Input: part model. Units: mm. Frame: model coordinates. A direction names the side the tool comes from. Give positions to 0.01 mm unless a question says otherwise; leave off trailing zeros. Order: outer loops, then holes, each group sorted by start corner. A loop starts at its lowest first (then second) coordinate and runs counter-clockwise, first axis right, second up. Notation, with made-up numbers: M 11.5,58.5 L 51.5,58.5 A35 cw 51.5,96.5 Z; hole C 82.5,39.25 d1. An arc over 180 degrees is marked long. Use a Markdown table: item, result.
from build123d import *

# Parameters (mm, degrees)
SKETCH4_R           = 2.54
BOSS_EXTRUDE1_DEPTH = 1.27
SKETCH5_W           = 12.7
SKETCH5_H           = 1.27
BOSS_EXTRUDE2_DEPTH = 28.956


with BuildPart() as part:
    # Sketch4 → Boss-Extrude1 (new body)
    with BuildSketch(Plane.XY):
        Polygon((0, 0), (12.7, 0), (12.7, 20.32), (9.525, 23.609765797), (3.175, 23.609765797), (0, 20.32), align=None)
        with Locations((6.35, 18.246144904)):
            Circle(SKETCH4_R, mode=Mode.SUBTRACT)
    boss_extrude1 = extrude(amount=BOSS_EXTRUDE1_DEPTH)

    # Sketch5 → Boss-Extrude2 (add)
    with BuildSketch(Plane.XY.offset(1.27)):
        with Locations((6.35, 0.635)):
            Rectangle(SKETCH5_W, SKETCH5_H)
    extrude(amount=BOSS_EXTRUDE2_DEPTH)

    # Mirror1: Boss-Extrude1 across plane
    add(boss_extrude1.mirror(Plane.XY.offset(15.113)))


solid = part.part
1) Cut plane D-D on y = 22. Return loops of the section in (x, z), and give its area (3 significant figures).
Response values:
| item | result |
|---|---|
| outline | M 1.62,0 L 11.08,0 L 11.08,1.27 L 1.62,1.27 Z; M 1.62,28.96 L 11.08,28.96 L 11.08,30.23 L 1.62,30.23 Z |
| area | 24.0 mm² |
2) First-contact query: pin 1 Ø1.5 at (x, z) = (5, 13.5) entering from +Y. Flat tip, straight axial feed; report the tip coordinate or a pass-through.
Response values:
| item | result |
|---|---|
| pin 1 | stops at y = 1.27 |
3) Cut plane C-C on z = 4.5. Return loops of the section in (x, y).
Response values:
| item | result |
|---|---|
| outline | M 0,0 L 12.7,0 L 12.7,1.27 L 0,1.27 Z |
4) Cut plane A-A on y = 7. Return loops of the section in (x, z), and give its area (3 significant figures).
Response values:
| item | result |
|---|---|
| outline | M 0,0 L 12.7,0 L 12.7,1.27 L 0,1.27 Z; M 0,28.96 L 12.7,28.96 L 12.7,30.23 L 0,30.23 Z |
| area | 32.3 mm² |
5) Mould query, pull axis Z, two halves, no side actions, for faces 3 (the face through (11.135, 21.942, 29.6)), 4 (the face through (6, 13, 1.27)), 5 (the face through (6, 12, 30.226)). Classes: released by +Z, released by -Z, zero draft, split by the parting line, or undercut.
Response values:
| item | result |
|---|---|
| face 3 | zero draft |
| face 4 | undercut |
| face 5 | released by +Z |
6) Material intervals for line 1 (Y direction, x = 6.35, z = 0.5); line 2 (Z direction, x = 11.25, y = 3); line 3 (Y direction, x = 10.5, z = 11.5), sorted ascending. Write a range as from..to.
Response values:
| item | result |
|---|---|
| line 1 | y = 0..15.71, 20.79..23.61 |
| line 2 | z = 0..1.27, 28.96..30.23 |
| line 3 | y = 0..1.27 |
7) Cut plane B-B on x = 6.35. Return loops of the section in (y, z), and give its area (3 significant figures).
Response values:
| item | result |
|---|---|
| outline | M 0,0 L 15.71,0 L 15.71,1.27 L 1.27,1.27 L 1.27,28.96 L 15.71,28.96 L 15.71,30.23 L 0,30.23 Z; M 20.79,0 L 23.61,0 L 23.61,1.27 L 20.79,1.27 Z; M 20.79,28.96 L 23.61,28.96 L 23.61,30.23 L 20.79,30.23 Z |
| area | 82.2 mm² |
8) Reachability of faces 1 (the face through (6, 1.27, 15)), 2 (the face through (1.61, 21.99, 29.6)) from +Z, -Z, +X, -X, +Y, -Y: full face, straight path, thin tool, end or side. Return the list, or none.
Response values:
| item | result |
|---|---|
| face 1 | +X, -X, +Y |
| face 2 | +Z, -Z, -X, +Y |
